from build123d import *

# Parameters (mm, degrees)
SALIENTE_EXTRUIR1_DEPTH = 5
CORTAR_EXTRUIR1_REACH   = 7
CROQUIS2_R              = 1.75
CROQUIS2_R_2            = 2.5
CROQUIS2_R_3            = 1.599246839
CROQUIS3_W              = 36.7
CROQUIS3_H              = 6.315423537
CORTAR_EXTRUIR2_DEPTH   = 10


with BuildPart() as part:
    # Croquis1 → Saliente-Extruir1 (new body)
    with BuildSketch(Plane(origin=(0, 0, 0), x_dir=(1, 0, 0), z_dir=(0, 1, 0))):
        Polygon((36, 0), (-36, 0), (-96.722621731, -28.315423537), (-96.722621731, -53.315423537), (96.722621731, -53.315423537), (96.722621731, -28.315423537), align=None)
    extrude(amount=SALIENTE_EXTRUIR1_DEPTH)

    # Croquis2 → Cortar-Extruir1 (cut, up to next)
    with BuildSketch(Plane(origin=(0, 5, 0), x_dir=(1, 0, 0), z_dir=(0, 1, 0)), mode=Mode.PRIVATE) as cortar_extruir1_sk1:
        with Locations((-84.339669031, -33.574937051)):
            Circle(CROQUIS2_R)
    cortar_extruir1_tool1 = extrude(cortar_extruir1_sk1.sketch, amount=-CORTAR_EXTRUIR1_REACH, mode=Mode.PRIVATE) & part.part
    add(cortar_extruir1_tool1.solids().sort_by_distance((-84.339669, 5, 33.574937))[0], mode=Mode.SUBTRACT)
    # Croquis2 → Cortar-Extruir1 (cut, up to next)
    with BuildSketch(Plane(origin=(0, 5, 0), x_dir=(1, 0, 0), z_dir=(0, 1, 0)), mode=Mode.PRIVATE) as cortar_extruir1_sk2:
        with Locations((-66.21351329, -25.122571817)):
            Circle(CROQUIS2_R)
    cortar_extruir1_tool2 = extrude(cortar_extruir1_sk2.sketch, amount=-CORTAR_EXTRUIR1_REACH, mode=Mode.PRIVATE) & part.part
    add(cortar_extruir1_tool2.solids().sort_by_distance((-66.213513, 5, 25.122572))[0], mode=Mode.SUBTRACT)
    # Croquis2 → Cortar-Extruir1 (cut, up to next)
    with BuildSketch(Plane(origin=(0, 5, 0), x_dir=(1, 0, 0), z_dir=(0, 1, 0)), mode=Mode.PRIVATE) as cortar_extruir1_sk3:
        with Locations((-55.648056746, -47.780266492)):
            Circle(CROQUIS2_R)
    cortar_extruir1_tool3 = extrude(cortar_extruir1_sk3.sketch, amount=-CORTAR_EXTRUIR1_REACH, mode=Mode.PRIVATE) & part.part
    add(cortar_extruir1_tool3.solids().sort_by_distance((-55.648057, 5, 47.780266))[0], mode=Mode.SUBTRACT)
    # Croquis2 → Cortar-Extruir1 (cut, up to next)
    with BuildSketch(Plane(origin=(0, 5, 0), x_dir=(1, 0, 0), z_dir=(0, 1, 0)), mode=Mode.PRIVATE) as cortar_extruir1_sk4:
        with Locations((-38.701346441, -39.877885696)):
            Circle(CROQUIS2_R)
    cortar_extruir1_tool4 = extrude(cortar_extruir1_sk4.sketch, amount=-CORTAR_EXTRUIR1_REACH, mode=Mode.PRIVATE) & part.part
    add(cortar_extruir1_tool4.solids().sort_by_distance((-38.701346, 5, 39.877886))[0], mode=Mode.SUBTRACT)
    # Croquis2 → Cortar-Extruir1 (cut, up to next)
    with BuildSketch(Plane(origin=(0, 5, 0), x_dir=(1, 0, 0), z_dir=(0, 1, 0)), mode=Mode.PRIVATE) as cortar_extruir1_sk5:
        with Locations((-43.555818614, -14.557115273)):
            Circle(CROQUIS2_R)
    cortar_extruir1_tool5 = extrude(cortar_extruir1_sk5.sketch, amount=-CORTAR_EXTRUIR1_REACH, mode=Mode.PRIVATE) & part.part
    add(cortar_extruir1_tool5.solids().sort_by_distance((-43.555819, 5, 14.557115))[0], mode=Mode.SUBTRACT)
    # Croquis2 → Cortar-Extruir1 (cut, up to next)
    with BuildSketch(Plane(origin=(0, 5, 0), x_dir=(1, 0, 0), z_dir=(0, 1, 0)), mode=Mode.PRIVATE) as cortar_extruir1_sk6:
        with Locations((38.868873457, -39.956004827)):
            Circle(CROQUIS2_R)
    cortar_extruir1_tool6 = extrude(cortar_extruir1_sk6.sketch, amount=-CORTAR_EXTRUIR1_REACH, mode=Mode.PRIVATE) & part.part
    add(cortar_extruir1_tool6.solids().sort_by_distance((38.868873, 5, 39.956005))[0], mode=Mode.SUBTRACT)
    # Croquis2 → Cortar-Extruir1 (cut, up to next)
    with BuildSketch(Plane(origin=(0, 5, 0), x_dir=(1, 0, 0), z_dir=(0, 1, 0)), mode=Mode.PRIVATE) as cortar_extruir1_sk7:
        with Locations((55.648056746, -47.780266492)):
            Circle(CROQUIS2_R)
    cortar_extruir1_tool7 = extrude(cortar_extruir1_sk7.sketch, amount=-CORTAR_EXTRUIR1_REACH, mode=Mode.PRIVATE) & part.part
    add(cortar_extruir1_tool7.solids().sort_by_distance((55.648057, 5, 47.780266))[0], mode=Mode.SUBTRACT)
    # Croquis2 → Cortar-Extruir1 (cut, up to next)
    with BuildSketch(Plane(origin=(0, 5, 0), x_dir=(1, 0, 0), z_dir=(0, 1, 0)), mode=Mode.PRIVATE) as cortar_extruir1_sk8:
        with Locations((84.339669031, -33.574937051)):
            Circle(CROQUIS2_R)
    cortar_extruir1_tool8 = extrude(cortar_extruir1_sk8.sketch, amount=-CORTAR_EXTRUIR1_REACH, mode=Mode.PRIVATE) & part.part
    add(cortar_extruir1_tool8.solids().sort_by_distance((84.339669, 5, 33.574937))[0], mode=Mode.SUBTRACT)
    # Croquis2 → Cortar-Extruir1 (cut, up to next)
    with BuildSketch(Plane(origin=(0, 5, 0), x_dir=(1, 0, 0), z_dir=(0, 1, 0)), mode=Mode.PRIVATE) as cortar_extruir1_sk9:
        with Locations((66.21351329, -25.122571817)):
            Circle(CROQUIS2_R)
    cortar_extruir1_tool9 = extrude(cortar_extruir1_sk9.sketch, amount=-CORTAR_EXTRUIR1_REACH, mode=Mode.PRIVATE) & part.part
    add(cortar_extruir1_tool9.solids().sort_by_distance((66.213513, 5, 25.122572))[0], mode=Mode.SUBTRACT)
    # Croquis2 → Cortar-Extruir1 (cut, up to next)
    with BuildSketch(Plane(origin=(0, 5, 0), x_dir=(1, 0, 0), z_dir=(0, 1, 0)), mode=Mode.PRIVATE) as cortar_extruir1_sk10:
        with Locations((43.555818614, -14.557115273)):
            Circle(CROQUIS2_R)
    cortar_extruir1_tool10 = extrude(cortar_extruir1_sk10.sketch, amount=-CORTAR_EXTRUIR1_REACH, mode=Mode.PRIVATE) & part.part
    add(cortar_extruir1_tool10.solids().sort_by_distance((43.555819, 5, 14.557115))[0], mode=Mode.SUBTRACT)
    # Croquis2 → Cortar-Extruir1 (cut, up to next)
    with BuildSketch(Plane(origin=(0, 5, 0), x_dir=(1, 0, 0), z_dir=(0, 1, 0)), mode=Mode.PRIVATE) as cortar_extruir1_sk11:
        with Locations((0, -10)):
            Circle(CROQUIS2_R_2)
    cortar_extruir1_tool11 = extrude(cortar_extruir1_sk11.sketch, amount=-CORTAR_EXTRUIR1_REACH, mode=Mode.PRIVATE) & part.part
    add(cortar_extruir1_tool11.solids().sort_by_distance((0, 5, 10))[0], mode=Mode.SUBTRACT)
    # Croquis2 → Cortar-Extruir1 (cut, up to next)
    with BuildSketch(Plane(origin=(0, 5, 0), x_dir=(1, 0, 0), z_dir=(0, 1, 0)), mode=Mode.PRIVATE) as cortar_extruir1_sk12:
        with Locations((0, -35)):
            Circle(CROQUIS2_R_2)
    cortar_extruir1_tool12 = extrude(cortar_extruir1_sk12.sketch, amount=-CORTAR_EXTRUIR1_REACH, mode=Mode.PRIVATE) & part.part
    add(cortar_extruir1_tool12.solids().sort_by_distance((0, 5, 35))[0], mode=Mode.SUBTRACT)
    # Croquis2 → Cortar-Extruir1 (cut, up to next)
    with BuildSketch(Plane(origin=(0, 5, 0), x_dir=(1, 0, 0), z_dir=(0, 1, 0)), mode=Mode.PRIVATE) as cortar_extruir1_sk13:
        with Locations((26, -10)):
            Circle(CROQUIS2_R)
    cortar_extruir1_tool13 = extrude(cortar_extruir1_sk13.sketch, amount=-CORTAR_EXTRUIR1_REACH, mode=Mode.PRIVATE) & part.part
    add(cortar_extruir1_tool13.solids().sort_by_distance((26, 5, 10))[0], mode=Mode.SUBTRACT)
    # Croquis2 → Cortar-Extruir1 (cut, up to next)
    with BuildSketch(Plane(origin=(0, 5, 0), x_dir=(1, 0, 0), z_dir=(0, 1, 0)), mode=Mode.PRIVATE) as cortar_extruir1_sk14:
        with Locations((26, -35)):
            Circle(CROQUIS2_R)
    cortar_extruir1_tool14 = extrude(cortar_extruir1_sk14.sketch, amount=-CORTAR_EXTRUIR1_REACH, mode=Mode.PRIVATE) & part.part
    add(cortar_extruir1_tool14.solids().sort_by_distance((26, 5, 35))[0], mode=Mode.SUBTRACT)
    # Croquis2 → Cortar-Extruir1 (cut, up to next)
    with BuildSketch(Plane(origin=(0, 5, 0), x_dir=(1, 0, 0), z_dir=(0, 1, 0)), mode=Mode.PRIVATE) as cortar_extruir1_sk15:
        with Locations((-26, -10)):
            Circle(CROQUIS2_R)
    cortar_extruir1_tool15 = extrude(cortar_extruir1_sk15.sketch, amount=-CORTAR_EXTRUIR1_REACH, mode=Mode.PRIVATE) & part.part
    add(cortar_extruir1_tool15.solids().sort_by_distance((-26, 5, 10))[0], mode=Mode.SUBTRACT)
    # Croquis2 → Cortar-Extruir1 (cut, up to next)
    with BuildSketch(Plane(origin=(0, 5, 0), x_dir=(1, 0, 0), z_dir=(0, 1, 0)), mode=Mode.PRIVATE) as cortar_extruir1_sk16:
        with Locations((-26, -35)):
            Circle(CROQUIS2_R_3)
    cortar_extruir1_tool16 = extrude(cortar_extruir1_sk16.sketch, amount=-CORTAR_EXTRUIR1_REACH, mode=Mode.PRIVATE) & part.part
    add(cortar_extruir1_tool16.solids().sort_by_distance((-26, 5, 35))[0], mode=Mode.SUBTRACT)

    # Croquis3 → Cortar-Extruir2 (cut)
    with BuildSketch(Plane(origin=(0, 5, 0), x_dir=(1, 0, 0), z_dir=(0, 1, 0))):
        with Locations((-0.941024734, -50.157711769)):
            Rectangle(CROQUIS3_W, CROQUIS3_H)
    extrude(amount=-CORTAR_EXTRUIR2_DEPTH, mode=Mode.SUBTRACT)


solid = part.part
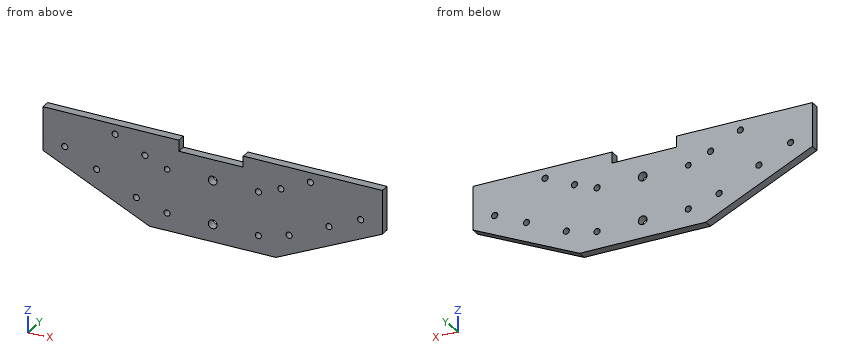
Here's how the part is built. I have some questions about the finished solid (model axes, mm). Coordinates: 2 decimals unless noted, no trailing zeros. Order: outer loops, then holes, each group sorted by start corner. A loop starts at its lowest first (then second) coordinate and runs counter-clockwise, first axis right, second up. Notation, with made-up numbers: (42, 35.5) - (98, 35.5) arc R25 cw to (98, 72.5) - close; hole circle Ø8 at (-32, 36.25). An arc over 180 degrees is marked (long way). Use CSV: the item, a comma, the result in double quotes. Start each with the question number.
1. Suppose I cut it at C-C on x = 0. List the corners of the cut face in (y, z) for me, then the cut area to 3 significant figures.
2. Suppose I cut it at A-A on x = 26. List the corners of the cut face in (y, z) for me.
3. Suppose I cut it at B-B on z = 10. List the corners of the cut face in (x, y) for me.
4. Please list where these lines run through material, in increasing order: line 1 (Z direction, x = 26, y = 3.95); line 2 (X direction, y = 3.2, z = 41); line 3 (X direction, y = 2, z = 35). Write a range as from..to.
5. I'm going to push flat-ended pins straight in: pin 1 (4.5 mm diameter, centred on x = 26, z = 35, fed in from +Y); pin 2 (1 mm diameter, centred on y = 4, z = 18, fed in from -X); pin 3 (1 mm diameter, centred on y = 4, z = 26, fed in from -X); pin 4 (2 mm diameter, centred on x = -57.5, y = 1, fed in from -Z). Where does each tip first touch, or does it pass through?
6. Suppose I cut it at D-D on y = 3.9. Give the number of separate pieces and of enclosed holes in the cut face, then the cut area to 3 significant figures.
Output:
1,outline,"(0, 0) - (5, 0) - (5, 7.5) - (0, 7.5) - close; (0, 12.5) - (5, 12.5) - (5, 32.5) - (0, 32.5) - close; (0, 37.5) - (5, 37.5) - (5, 47) - (0, 47) - close"
1,area,"185 mm2"
2,outline,"(0, 0) - (5, 0) - (5, 8.25) - (0, 8.25) - close; (0, 11.75) - (5, 11.75) - (5, 33.25) - (0, 33.25) - close; (0, 36.75) - (5, 36.75) - (5, 53.32) - (0, 53.32) - close"
3,outline,"(-57.45, 0) - (-27.75, 0) - (-27.75, 5) - (-57.45, 5) - close; (-24.25, 0) - (-2.5, 0) - (-2.5, 5) - (-24.25, 5) - close; (2.5, 0) - (24.25, 0) - (24.25, 5) - (2.5, 5) - close; (27.75, 0) - (57.45, 0) - (57.45, 5) - (27.75, 5) - close"
4,line 1,"z = 0..8.25, 11.75..33.25, 36.75..53.32"
4,line 2,"x = -96.72..-40.04, -37.36..37.46, 40.27..96.72"
4,line 3,"x = -96.72..-85.36, -83.32..-27.6, -24.4..-2.5, 2.5..24.25, 27.75..83.32, 85.36..96.72"
5,pin 1,"stops at y = 5"
5,pin 2,"stops at x = -75.67"
5,pin 3,"stops at x = -92.83"
5,pin 4,"stops at z = 9.56"
6,separate pieces,"1"
6,enclosed holes,"16"
6,area,"8,190 mm2"
